from build123d import *

# Parameters (mm, degrees)
ESQUISSE1_R        = 1.75
BOSS_EXTRU_1_DEPTH = 3
ESQUISSE1_3_W      = 13
ESQUISSE1_3_H      = 15
ESQUISSE1_3_W_2    = 7
ESQUISSE1_3_H_2    = 9
BOSS_EXTRU_2_DEPTH = 13
NERVURE2_REACH     = 30.623
ESQUISSE5_WALL_W   = 70.657799336
ESQUISSE5_WALL_H   = 3
ESQUISSE1_4_W      = 7
ESQUISSE1_4_H      = 9
BOSS_EXTRU_3_DEPTH = 7.5


with BuildPart() as part:
    # Esquisse1 → Boss.-Extru.1 (new body)
    with BuildSketch(Plane.XY):
        Polygon((-6.5, -7.5), (-6.5, 7.5), (4, 7.5), (4, 15), (-12, 15), (-12, -15), (4, -15), (4, -7.5), align=None)
        with Locations((-9.25, 0)):
            Circle(ESQUISSE1_R, mode=Mode.SUBTRACT)
        with Locations((-4, 12.5)):
            Circle(ESQUISSE1_R, mode=Mode.SUBTRACT)
        with Locations((-4, -12.5)):
            Circle(ESQUISSE1_R, mode=Mode.SUBTRACT)
    extrude(amount=BOSS_EXTRU_1_DEPTH)

    # Esquisse1_3 → Boss.-Extru.2 (add)
    with BuildSketch(Plane.XY):
        Rectangle(ESQUISSE1_3_W, ESQUISSE1_3_H)
        Rectangle(ESQUISSE1_3_W_2, ESQUISSE1_3_H_2, mode=Mode.SUBTRACT)
    extrude(amount=BOSS_EXTRU_2_DEPTH)

    # Esquisse5 wall → Nervure2 (add, up to next)
    with BuildSketch(Plane(origin=(-9.25, -7.5, 8), x_dir=(-0.481918749772, 0, -0.876215908677), z_dir=(0.876215908677, 0, -0.481918749772)), mode=Mode.PRIVATE) as nervure2_sk1:
        with Locations((0, 1.5)):
            Rectangle(ESQUISSE5_WALL_W, ESQUISSE5_WALL_H)
    nervure2_tool1 = extrude(nervure2_sk1.sketch, amount=NERVURE2_REACH, mode=Mode.PRIVATE) - part.part
    nervure2 = nervure2_tool1.solids().sort_by_distance((-9.25, -7.5, 8))[0]
    add(nervure2)

    # Sym_trie4: Nervure2 across plane
    add(nervure2.mirror(Plane.ZX))

    # Esquisse1_4 → Boss.-Extru.3 (add)
    with BuildSketch(Plane.XY):
        Rectangle(ESQUISSE1_4_W, ESQUISSE1_4_H)
    extrude(amount=BOSS_EXTRU_3_DEPTH)


solid = part.part
The model under review builds one solid part; all positions refer to its coordinate system, in mm. A direction names the side the tool comes from. Coordinates: 2 decimals unless noted, no trailing zeros. Loops run counter-clockwise (first coordinate to the right, second up) from the corner with the lowest first, then second, coordinate; pieces in that order, holes last. Notation, with made-up numbers: M 24.25,33 L 77.25,33 A20 ccw 77.25,48 Z; hole C 79.25,-28 d2. An arc over 180 degrees is marked long. Put each result on its own line as item: value. Start each with the question number.
Q1. Wall thickness on line 1 (Y direction, x = -4, z = 1.6); line 2 (Y direction, x = -10.25, z = 5.75); line 3 (X direction, y = -4.25, z = 8.5): over which ranges is each line inside the solid? List them lowest first.
Q2. Add section A-A (y = 12.5). Write out the cut boundary in (x, z), and give its area (3 significant figures).
Q3. The part is to be moulded in two halves that separate along Y. For faces 5 (the flat face through (-4, -15, 1)), 6 (the cylindrical face through (-5.29, -11.32, 1.48)), 7 (the flat face through (-3, 0, 0)), say which applies: +Y half, -Y half, draft (parallel to the pull), parting line (faces both ways), or undercut.
Q4. Clearance check with flat-ended pins moving along their axes: pin 1 (1.6 mm diameter, centred on x = -1.5, z = 10.5, fed in from -Y); pin 2 (0.9 mm diameter, centred on y = -11, z = 1, fed in from +X); pin 3 (2.5 mm diameter, centred on x = -10.5, z = 10, fed in from +Y); pin 4 (3.5 mm diameter, centred on x = -1, y = 0.5, fed in from +Z). State where each tip first meets the part, or that it passes through.
Q5. Add section B-B (x = -4). Write out the cut boundary in (y, z), and give its area (3 significant figures).
Q6. For faces 1 (the flat face through (4, 11, 1)), 2 (the flat face through (-4, -10, 3)), 3 (the flat face through (-9, 4.5, 6)), 4 (the flat face through (0, 4.5, 10)), list the 3-axis set-ups (+Z, -Z, +X, -X, +Y, -Y) from which the entire face can be reached by the end or side of a thin tool; tool diameter is ignored.
Q7. Add section D-D (x = -9.25). Write out the cut boundary in (y, z).
Q8. Add section C-C (z = 12). Write out the cut boundary in (x, y), and give its area (3 significant figures).
Answers:
1. line 1: y = -15 to -14.25, -10.75 to 10.75, 14.25 to 15
1. line 2: y = -7.5 to -4.5, 4.5 to 7.5
1. line 3: x = -6.5 to -3.5, 3.5 to 6.5
2. outline: M -12,0 L -5.75,0 L -5.75,3 L -12,3 Z; M -2.25,0 L 4,0 L 4,3 L -2.25,3 Z
2. area: 37.5 mm^2
3. face 5: -Y half
3. face 6: undercut
3. face 7: draft
4. pin 1: stops at y = -7.5
4. pin 2: stops at x = 4
4. pin 3: passes through
4. pin 4: stops at z = 7.5
5. outline: M -15,0 L -14.25,0 L -14.25,3 L -15,3 Z; M -10.75,0 L 10.75,0 L 10.75,3 L 7.5,3 L 7.5,13 L -7.5,13 L -7.5,3 L -10.75,3 Z; M 14.25,0 L 15,0 L 15,3 L 14.25,3 Z
5. area: 219 mm^2
6. face 1: +Z, -Z, +X, +Y
6. face 2: +Z, +X, -X, -Y
6. face 3: +Z, -X
6. face 4: +Z
7. outline: M -15,0 L -1.75,0 L -1.75,3 L -4.5,3 L -4.5,8 L -7.5,8 L -7.5,3 L -15,3 Z; M 1.75,0 L 15,0 L 15,3 L 7.5,3 L 7.5,8 L 4.5,8 L 4.5,3 L 1.75,3 Z
8. outline: M -7.05,-7.5 L 6.5,-7.5 L 6.5,7.5 L -7.05,7.5 L -7.05,4.5 L -6.5,4.5 L -6.5,-4.5 L -7.05,-4.5 Z; hole M -3.5,-4.5 L 3.5,-4.5 L 3.5,4.5 L -3.5,4.5 Z
8. area: 135 mm^2
